```python
from build123d import *

# Parameters (mm, degrees)
BASE_FLANGE1_DEPTH     = 6
SKETCHED_START         = -25
SKETCHED_BEND1_DEPTH   = 50
SKETCHED_BEND1_2_DEPTH = 50
SKETCH8_R              = 3
CUT_EXTRUDE1_DEPTH     = 82.299658022
SKETCH9_R              = 3
CUT_EXTRUDE2_DEPTH     = 88.83868393
FILLET1_R              = 10


# Read off the part's stored shape, not the designer's step: Sketched Bend1
# Sheet-metal steps are written as plain solids
with BuildPart() as part:
    # Sketch1 → Base-Flange1 (new body)
    with BuildSketch(Plane(origin=(0, 0, 0), x_dir=(1, 0, 0), z_dir=(0, 1, 0))):
        Polygon((25, 20), (67.5, 20), (67.5, -20), (-67.5, -20), (-67.5, 20), (-25, 20), (-25, 60), (25, 60), align=None)
    extrude(amount=-BASE_FLANGE1_DEPTH)

    # Sketched Bend1 outline → Sketched Bend1 (cut)
    with BuildSketch(Plane.YZ.offset(SKETCHED_START)):
        with BuildLine():
            Line((0, -60), (0, -30.677078252))
            ThreePointArc((0, -30.677078252), (-4.397247359, -26.123724357), (-6, -20))
            Line((-6, -20), (-6, -60))
            Line((-6, -60), (0, -60))
        make_face()
    extrude(amount=SKETCHED_BEND1_DEPTH, mode=Mode.SUBTRACT)

    # Sketched Bend1 2 outline → Sketched Bend1 2 (add)
    with BuildSketch(Plane.YZ.offset(SKETCHED_START)):
        with BuildLine():
            Line((6.5, -32.5), (31.577434895, -32.5))
            Line((31.577434895, -32.5), (31.577434895, -26.5))
            Line((31.577434895, -26.5), (6.5, -26.5))
            ThreePointArc((6.5, -26.5), (1.903805922, -24.596194078), (0, -20))
            Line((0, -20), (0, -30.677078252))
            ThreePointArc((0, -30.677078252), (3.124609515, -32.035644523), (6.5, -32.5))
        make_face()
    extrude(amount=SKETCHED_BEND1_2_DEPTH)

    # Sketch8 → Cut-Extrude1 (cut, through all)
    with BuildSketch(Plane(origin=(0, 0, 0), x_dir=(1, 0, 0), z_dir=(0, 1, 0))):
        with Locations(Location((-55, -7.5, 0), (0, 0, 270))):
            Circle(SKETCH8_R)
        with Locations(Location((55, -7.5, 0), (0, 0, 90))):
            Circle(SKETCH8_R)
    extrude(amount=-CUT_EXTRUDE1_DEPTH, mode=Mode.SUBTRACT)

    # Sketch9 → Cut-Extrude2 (cut, through all)
    with BuildSketch(Plane.XY.offset(-26.5)):
        with Locations((-7.5, 21.577434895)):
            Circle(SKETCH9_R)
        with Locations(Location((7.5, 21.577434895, 0), (0, 0, 180))):
            Circle(SKETCH9_R)
    extrude(amount=-CUT_EXTRUDE2_DEPTH, mode=Mode.SUBTRACT)

    # Fillet1
    fillet1_edges = [part.edges().sort_by_distance(p)[0] for p in [
        (-67.5, -3, 20),
        (67.5, -3, 20),
        (67.5, -3, -20),
        (-67.5, -3, -20),
    ]]
    fillet(fillet1_edges, radius=FILLET1_R)


solid = part.part
```
For this review, take the finished solid that the model builds, in its own axes (mm). A direction names the side the tool comes from. Coordinates: 2 decimals unless noted, no trailing zeros. Loops run counter-clockwise (first coordinate to the right, second up) from the corner with the lowest first, then second, coordinate; pieces in that order, holes last. Notation, with made-up numbers: (87.25, 44) -> (95.25, 44) arc R24 cw to (95.25, 72) -> close; hole circle Ø7 at (7.5, -15.75). An arc over 180 degrees is marked (long way). Return JSON: item names as keys, results as strings. Group by question number.
(1) Consider section B-B, the plane x = -55. Give the boundary of the cut face in (y, z).
(2) To check wall thickness, follow L1, parallel to X at y = -1.65, z = 7.5; L2, parallel to Z at x = 55, y = -2.95; L3, parallel to Y at x = -11.5, z = 8. State the ranges of each line that lie inside material, in increasing order.
(3) For pin 1 Ø14 at (y, z) = (18.5, -23.5) entering from +X; pin 2 Ø3.5 at (x, z) = (-55, 7.5) entering from +Y; pin 3 Ø5 at (x, z) = (-10.5, 3.5) entering from +Y; pin 4 Ø7 at (x, y) = (7.5, 21.58) entering from +Z, all flat-tipped, find the tip position at first contact; note any pin that passes through.
(4) Consider section A-A, the plane z = 7.5. Give the boundary of the cut face in (x, y).
(5) Consider section D-D, the plane x = 7.5. Give the boundary of the cut face in (y, z).
(6) Consider section C-C, the plane y = 20. Give the boundary of the cut face in (x, z).
(7) Tool access review of faces 1 (the flat face through (-25, 13, -28)), 2 (the cylindrical face through (-5.89, 24.11, -29.46)), 3 (the flat face through (25, 13, -28)), 4 (the flat face through (1, 0, 0)): name each direction out of +Z, -Z, +X, -X, +Y, -Y from which nothing blocks a thin tool from reaching the whole face with its end or side.
(8) Mouldability with a two-part tool opening along Z and no side actions: class faces 5 (the cylindrical face through (-52.47, -2.96, 9.11)), 6 (the flat face through (-67.5, -3, 0)), 7 (the cylindrical face through (-64.65, -3.04, 16.99)), 8 (the cylindrical face through (52.47, -2.96, 5.89)) as pulls with the +Z half, pulls with the -Z half, needs draft (parallel to the pull), parting line crosses it, or undercut.
Results below:
{
 "1": {"outline": "(-6, -20) -> (0, -20) -> (0, 4.5) -> (-6, 4.5) -> close; (-6, 10.5) -> (0, 10.5) -> (0, 20) -> (-6, 20) -> close"},
 "2": {"L1": "x = -67.5 to -58, -52 to 52, 58 to 67.5", "L2": "z = -20 to 4.5, 10.5 to 20", "L3": "y = -6 to 0"},
 "3": {"pin 1": "stops at x = 25", "pin 2": "passes through", "pin 3": "stops at y = 0", "pin 4": "stops at z = -26.5"},
 "4": {"outline": "(-67.5, -6) -> (-58, -6) -> (-58, 0) -> (-67.5, 0) -> close; (-52, -6) -> (52, -6) -> (52, 0) -> (-52, 0) -> close; (58, -6) -> (67.5, -6) -> (67.5, 0) -> (58, 0) -> close"},
 "5": {"outline": "(-6, -20) arc R12.5 ccw to (6.5, -32.5) -> (18.58, -32.5) -> (18.58, -26.5) -> (6.5, -26.5) arc R6.5 cw to (0, -20) -> (0, 20) -> (-6, 20) -> close; (24.58, -32.5) -> (31.58, -32.5) -> (31.58, -26.5) -> (24.58, -26.5) -> close"},
 "6": {"outline": "(-25, -32.5) -> (-10.05, -32.5) -> (-10.05, -26.5) -> (-25, -26.5) -> close; (-4.95, -32.5) -> (4.95, -32.5) -> (4.95, -26.5) -> (-4.95, -26.5) -> close; (10.05, -32.5) -> (25, -32.5) -> (25, -26.5) -> (10.05, -26.5) -> close"},
 "7": {"face 1": "-Z, -X, +Y, -Y", "face 2": "+Z, -Z", "face 3": "-Z, +X, +Y, -Y", "face 4": "+Z, +X, -X, +Y"},
 "8": {"face 5": "undercut", "face 6": "needs draft", "face 7": "pulls with the +Z half", "face 8": "undercut"}
}
